Geometry: final body of the model. Coordinates: model frame, mm. A direction names the side the tool comes from. Coordinates: 2 decimals unless noted, no trailing zeros. Loops run counter-clockwise (first coordinate to the right, second up) from the corner with the lowest first, then second, coordinate; pieces in that order, holes last. Notation, with made-up numbers: (54.25, 67.25) - (67.25, 67.25) arc R16 ccw to (67.25, 97.25) - close; hole circle Ø5 at (-1.75, -37.75). An arc over 180 degrees is marked (long way). Write each question's results on one line, items separated by ' | '. Start each with the question number.
Autodesk Inventor part; units mm, degrees
ref_plane "Work Plane3" through (0, 16.5, 0) normal (0, -1, 0) x (1, 0, 0)
ref_plane "YZ Plane" through (0, 0, 0) normal (1, 0, 0) x (0, 1, 0)
ref_plane "XZ Plane" through (0, 0, 0) normal (0, 1, 0) x (-1, 0, 0)
sketch "Base Profile" plane through (0, 0, 0) normal (0, 1, 0) x (-1, 0, 0)
  line L0 (0, 0) -> (-15, 0)
  line L1 (-15, 0) -> (-15, -13)
  line L2 (-15, -13) -> (0, -13)
  line L3 (0, -13) -> (0, 0)
  line L4 (-15, -13) -> (-21.35, -13)
  line L5 (-21.35, -13) -> (-21.35, 0)
  line L6 (-21.35, 0) -> (-15, 0)
  line L7 (-7.5, -13) -> (-7.5, 0) construction
  circle A0 centre (-7.5, -6.5) radius 1.5
  line L8 (-6, -13) -> (-6, 0)
  line L9 (-9, -13) -> (-9, 0)
  circle A1 centre (-7.5, -6.5) radius 3.175
  point P0 (-9, 0)
  dimension "d376" = 15
  dimension "d380" = 13
  dimension "d381" = 6.35
  dimension "d395" = 3
  dimension "d405" = 6.35
extrude "Stock" add sketch "Base Profile" along normal blind 33
ref_plane "Work Plane3" through (0, 16.5, 0) normal (0, -1, 0) x (1, 0, 0)
extrude "Guide" add sketch "Base Profile" against normal blind 3 contours L8 A1 L9 L0 | L8 A0 L9 A1 | L2 L9 A1 L8 | A0 | L8 A1 L9 A0
mirror "Mirror3" about plane through (0, 16.5, 0) normal (0, -1, 0) of "Guide"
sketch "Front Profile" plane through (0, 0, 0) normal (0, 0, 1) x (1, 0, 0)
  line L0 (21.35, 0) -> (21.35, 33)
  line L1 (0, 33) -> (6, 33)
  line L2 (0, 0) -> (0, 33)
  line L3 (0, 16.5) -> (21.35, 16.5)
  line L4 (0, 7.5) -> (21.35, 7.5)
  line L5 (15, 33) -> (15, 0)
  line L6 (9, 0) -> (21.35, 0)
  line L7 (0, 0) -> (6, 0)
  line L8 (6, 0) -> (6, -3)
  line L9 (9, -3) -> (6, -3)
  line L10 (9, 0) -> (9, -3)
  line L11 (9, 33) -> (21.35, 33)
  line L12 (9, 33) -> (9, 36)
  line L13 (9, 36) -> (6, 36)
  line L14 (6, 33) -> (6, 36)
  line L15 (15, 24) -> (21.35, 24)
  line L16 (15, 16.5) -> (21.35, 24) construction
  line L17 (21.35, 7.5) -> (15, 0) construction
  circle A0 centre (18.175, 20.25) radius 1.5
  circle A1 centre (18.175, 3.75) radius 1.5
  point P0 (15, 7.5)
  dimension "d383" = 9
  dimension "d384" = 6.35
  dimension "d408" = 7.5
  dimension "d409" = 7.5
  dimension "d413" = 3
  dimension "d414" = 3
extrude "Bearing Clearance" cut sketch "Front Profile" against normal through all contours L4 L2 L3 L5
extrude "Hole Clearance" cut sketch "Base Profile" against normal blind 3 from surface at 36 contours A1 L8 | L8 A0 L9 A1 | L9 A1 | A0 | L8 A1 L9 A0
hole "Hole25" at (7.5, 0, -6.5) direction (0, 1, 0) diameter 3 end through all
extrude "Extrusion22" cut sketch "Front Profile" against normal through all contours L15 L5 L11 L0
fillet "Fillet3" radius 3.175 2 edges at (21.35, 24, -6.5) (21.35, 0, -6.5)
hole "Hole26" at (18.175, 20.25, 0) at (18.175, 3.75, 0) direction (0, 0, -1) diameter 2.459 end through all
equation "\"extrusionWidth\" = 15"
equation "\"idlerLength\" = 0"
equation "\"bearingOffsetFromBottom\" = 7.5"
equation "\"extrusionOffset\" = 33"
equation "\"d165\" = extrusionWidth"
equation "\"bearingStackHeight\" = 9"
equation "\"bearingSlotLength\" = 0"
equation "\"bearingClearance\" = 13"
equation "\"pinSupportLength\" = 2"
properties part number "B Idler (Tulip)" material "Aluminum 6061"
1) Section query A-A on y = 3.75. Output: boundary loops of the cut face in (x, z).
2) Pull-direction query (Z, two-part tool) for faces 6 (the flat face through (17, 24, -6)), 7 (the flat face through (11, 21, -13)), 8 (the cylindrical face through (8.4, 24.9, -5.3)); classes: released by +Z, released by -Z, zero draft, split by the parting line, or undercut.
3) Material intervals for line 1 (Z direction, x = 7.5, y = 29); line 2 (Y direction, x = 4, z = -8.5); line 3 (Y direction, x = 19, z = -10.25), sorted ascending. Write a range as [from, to].
4) Section query B-B on x = 7.5. Output: boundary loops of the cut face in (y, z) (3 decimals), and give its area (3 significant figures).
5) Access query for faces 1 (the flat face through (9, 34, -11)), 2 (the flat face through (5.7, 7.5, -6.4)), 3 (the flat face through (6, 34, -2)), 4 (the flat face through (9, -1, -7)), 5 (the cylindrical face through (7.478, 34.521, -3.325)). Directions: +Z, -Z, +X, -X, +Y, -Y. A direction counts if a zero-diameter tool reaches every point of the face in a straight line with its end or side. Return the directions, or none.
6) Pin query (flat end, axial travel): pin 1 Ø4.5 at (y, z) = (27.5, -4) entering from +X; pin 2 Ø3.5 at (x, z) = (8, -6.5) entering from +Y; pin 3 Ø1.5 at (y, z) = (34, -2.5) entering from -X. Return the tip coordinate at first contact, or that it passes through.
7) Section query C-C on z = -2. Count the separate pieces of the cut face and the enclosed holes in it, and give its area (3 significant figures).
8) Section query D-D on y = 28.5. Output: boundary loops of the cut face in (x, z).
Returned:
1) outline: (0, -13) - (16.95, -13) - (16.95, 0) - (0, 0) - close; (19.4, -13) - (21.35, -13) - (21.35, 0) - (19.4, 0) - close; hole circle Ø3 at (7.5, -6.5)
2) face 6: zero draft | face 7: released by -Z | face 8: undercut
3) line 1: z = [-13, -8], [-5, 0] | line 2: y = [0, 7.5], [16.5, 33] | line 3: y = [0.11, 2.84], [4.66, 19.34], [21.16, 23.89]
4) outline: (-3, -13) - (7.5, -13) - (7.5, -8) - (0, -8) - (0, -5) - (7.5, -5) - (7.5, 0) - (-3, 0) - close; (16.5, -13) - (36, -13) - (36, -9.675) - (33, -9.675) - (33, -8) - (16.5, -8) - close; (16.5, -5) - (33, -5) - (33, -3.325) - (36, -3.325) - (36, 0) - (16.5, 0) - close | area: 299 mm²
5) face 1: +Z, -Z, +X, +Y | face 2: +Z, -Z, -X | face 3: +Z, -Z, -X, +Y | face 4: +Z, -Z, +X, -Y | face 5: +Y
6) pin 1: stops at x = 15 | pin 2: stops at y = 33 | pin 3: stops at x = 6
7) separate pieces: 1 | enclosed holes: 2 | area: 517 mm²
8) outline: (0, -13) - (15, -13) - (15, 0) - (0, 0) - close; hole circle Ø3 at (7.5, -6.5)
